Input: part model. Units: mm. Frame: model coordinates. Round coordinates to 2 decimals unless told otherwise and drop trailing zeros. Write each loop counter-clockwise with the first axis right and the second up, starting at its lowest first coordinate (ties: lowest second). Pieces come first, ordered by that corner, then holes. Notation, with made-up numbers: (50, 5) - (72, 5) arc R16 cw to (72, 31) - close; hole circle Ø2 at (42.5, 59.25). An arc over 180 degrees is marked (long way). Use one line per item in the form item = value.
```python
from build123d import *

# Parameters (mm, degrees)
F0_R     = 38.1
F1_DEPTH = 91.44
F2_R     = 23.1008347908
F3_DEPTH = 25.4
F4_R     = 5.08


with BuildPart() as f1:
    # F0 (on Front) → F1 (new body)
    with BuildSketch(Plane.XZ):
        Circle(F0_R)
    extrude(amount=F1_DEPTH)

    # F2 (on face) → F3 (cut)
    with BuildSketch(Plane.XZ.offset(91.44)):
        Circle(F2_R)
    extrude(amount=-F3_DEPTH, mode=Mode.SUBTRACT)

    # F4
    f4_edges = [f1.edges().sort_by_distance(p)[0] for p in [
        (-38.1, -91.44, 0),
    ]]
    fillet(f4_edges, radius=F4_R)

    # F5 (on Top) → F6 (revolve)
    with BuildSketch(Plane.XY):
        with BuildLine():
            Line((0, 68.6084377315), (0, 0))
            Line((0, 0), (38.1, 0))
            add(Edge.make_bspline(
                [(0, 68.6084377315), (6.2479440962, 66.531043979), (20.3802893777, 61.8529112655), (20.0334067384, 35.4150108531), (23.0129778355, 17.0896280583), (35.4184549534, 4.6880386636), (38.1, 0)],
                knots=[0, 0, 0, 0, 0.238836495, 0.5037885419, 0.7463651992, 1, 1, 1, 1], degree=3))
        make_face()
    revolve(axis=Axis((0, 34.3042188658, 0), (0, 1, 0)))


solid = f1.part
```
(1) Material intervals for L1, parallel to Z at x = 0, y = -71; L2, parallel to Z at x = 27.5, y = -30; L3, parallel to X at y = 15, z = -23, sorted ascending.
Derived:
L1 = -38.1 to -23.1, 23.1 to 38.1
L2 = -26.37 to 26.37
L3 = -13.91 to 13.91
(2) Cut plane A-A on y = -53. Output: boundary loops of the cut face in (x, z), then the cut area to 3 significant figures.
Derived:
outline = circle Ø76.2 at (0, 0)
area = 4,560 mm^2
(3) Draft query along X for faces 1 (the face through (0, -66.04, 0)), 2 (the face through (-22.5, -91.44, -6.9)), 3 (the face through (-30.235, -42.575, -23.183)). Return one class per face: released by +X, released by -X, zero draft, split by the parting line, or undercut.
Derived:
face_1 = undercut
face_2 = zero draft
face_3 = split by the parting line
(4) First-contact query: pin 1 Ø1.5 at (x, y) = (-14, 29) entering from -Z; pin 2 Ø1 at (x, y) = (17.5, -52) entering from -Z; pin 3 Ø6 at (y, z) = (-64, 7.5) entering from -X. Flat tips, straight axial feed; report the tip coordinate or a pass-through.
Derived:
pin_1 = -16.8
pin_2 = -34.1
pin_3 = -37.83
